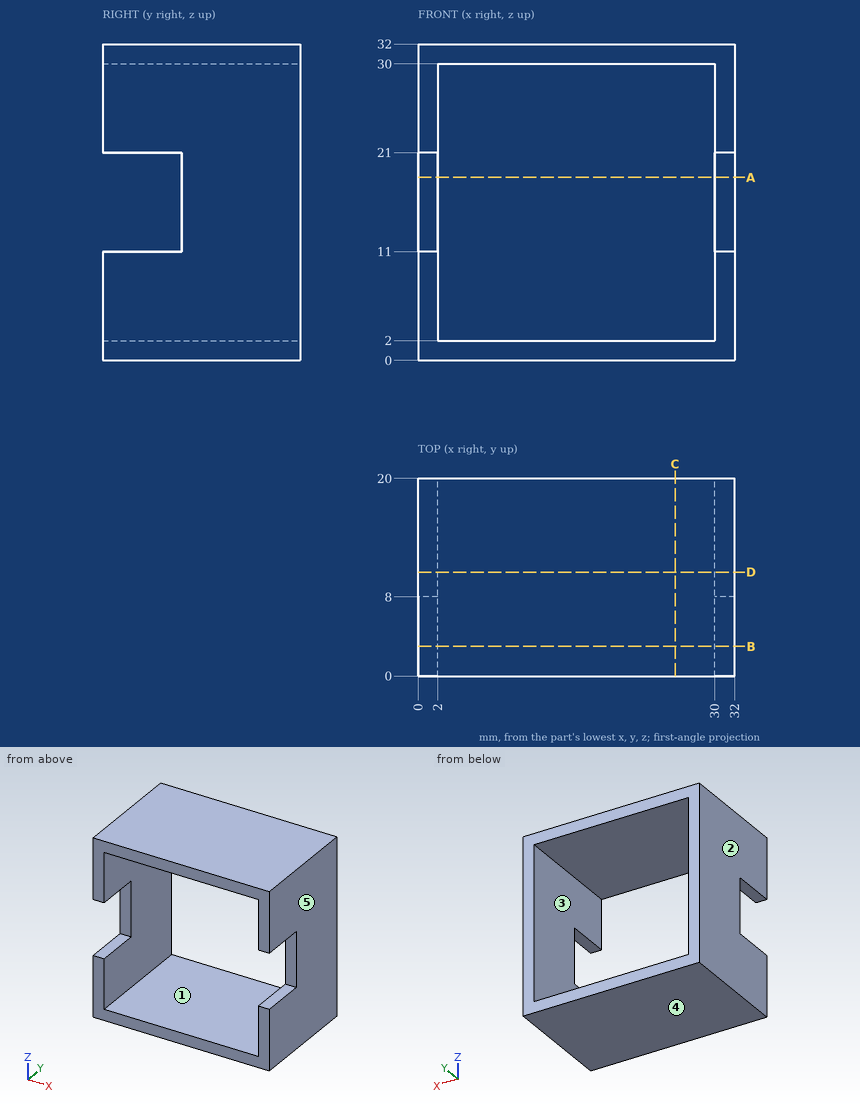
Design review of the part shown in the three views and the two pictorial views. Dimensions are in mm from the part's minimum x, y and z. A direction names the side the tool comes from. Give positions to 0.01 mm unless a question says otherwise; leave off trailing zeros. Loops run counter-clockwise (first coordinate to the right, second up) from the corner with the lowest first, then second, coordinate; pieces in that order, holes last. Notation, with made-up numbers: M -40,-15 L 13,-15 A29 cw 13,12 Z; hole C 75.25,-24.75 d10. An arc over 180 degrees is marked long. Answer as a JSON object with one key per item and string values.
Item 1: We need section C-C (x = 26). State the section outline as (y, z) points, and give its area (3 significant figures).
Output values:
{"outline": "M 0,0 L 20,0 L 20,2 L 0,2 Z; M 0,30 L 20,30 L 20,32 L 0,32 Z", "area": "80.0 mm2"}
Item 2: We need section D-D (y = 10.5). State the section outline as (x, z) points.
Output values:
{"outline": "M 0,0 L 32,0 L 32,32 L 0,32 Z; hole M 2,2 L 30,2 L 30,30 L 2,30 Z"}
Item 3: We need section B-B (y = 3). State the section outline as (x, z) points, and give its area (3 significant figures).
Output values:
{"outline": "M 0,0 L 32,0 L 32,11 L 30,11 L 30,2 L 2,2 L 2,11 L 0,11 Z; M 0,21 L 2,21 L 2,30 L 30,30 L 30,21 L 32,21 L 32,32 L 0,32 Z", "area": "200 mm2"}
Item 4: For P1, Ø0.6, axis at x = 31, z = 18, coming from the -Y side, flat-tipped, find the tip position at first contact; note if it passes through.
Output values:
{"P1": "stops at y = 8"}
Item 5: We need section A-A (z = 18.5). State the section outline as (x, y) points, and give its area (3 significant figures).
Output values:
{"outline": "M 0,8 L 2,8 L 2,20 L 0,20 Z; M 30,8 L 32,8 L 32,20 L 30,20 Z", "area": "48.0 mm2"}
Item 6: Wall thickness on line 1 along Z through (x, y) = (3.5, 13.25); line 2 along Z through (x, y) = (31.5, 6.25): over which ranges is each line inside the solid? List them lowest first.
Output values:
{"line 1": "z = 0 to 2, 30 to 32", "line 2": "z = 0 to 11, 21 to 32"}
Item 7: Mouldability with a two-part tool opening along X and no side actions: class the marked faces 3, 4 and 5 as pulls with the +X half, pulls with the -X half, needs draft (parallel to the pull), parting line crosses it, or undercut.
Output values:
{"face 3": "undercut", "face 4": "needs draft", "face 5": "pulls with the +X half"}
Item 8: Machinability: for the marked faces 1 and 2, which of the approach directions +Z, -Z, +X, -X, +Y, -Y give a long, thin tool a straight path to every point of the face, cutting with its end or side? Answer none if there is none.
Output values:
{"face 1": "+Y, -Y", "face 2": "+Z, -Z, -X, +Y, -Y"}
